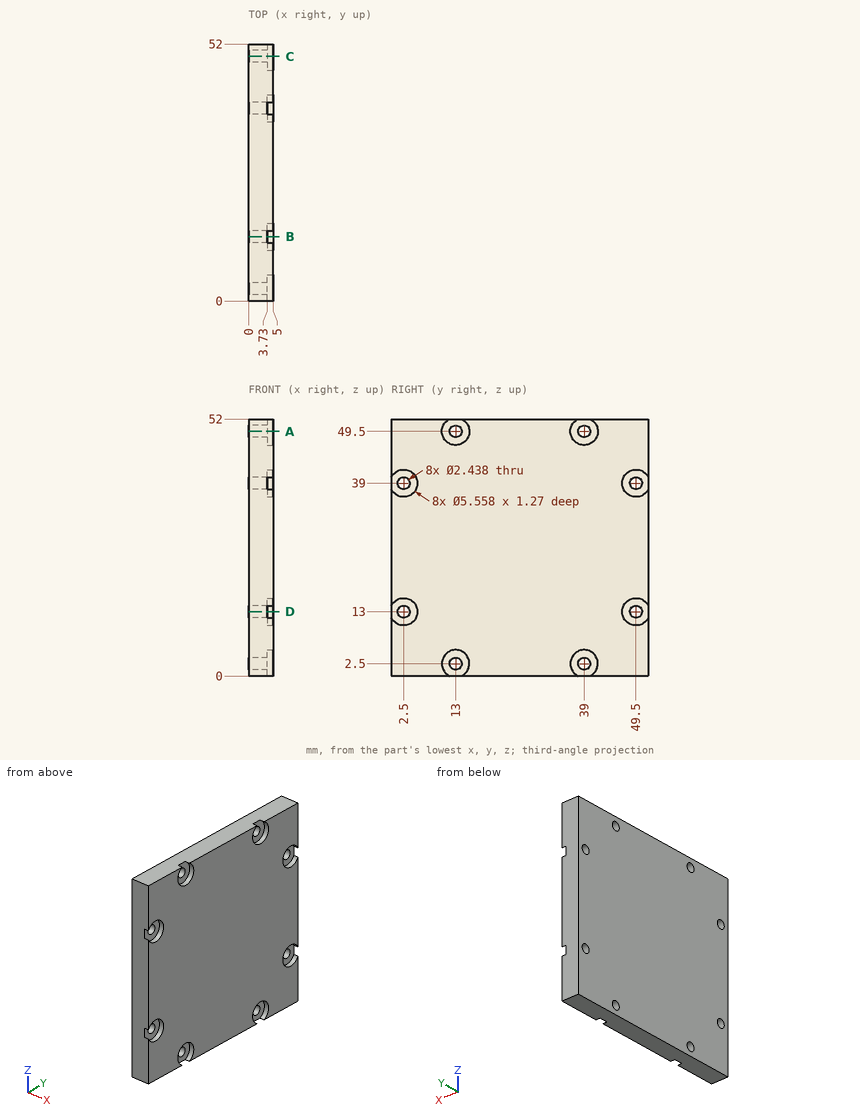
Drawing for the job (mm, zero at the part's lowest x, y, z). Give positions to 0.01 mm unless a question says otherwise; leave off trailing zeros. Order: outer loops, then holes, each group sorted by start corner. A loop starts at its lowest first (then second) coordinate and runs counter-clockwise, first axis right, second up. Notation, with made-up numbers: M 18,37 L 44,37 A6 ccw 44,48 Z; hole C -24,35 d8. An arc over 180 degrees is marked long. Put each result on its own line as item: value.
Item 1: Probe line 1 (Y direction, x = 1.1, z = 49.5); line 2 (Y direction, x = 4.3, z = 36.5) (1 decimal); line 3 (Z direction, x = 4.7, y = 2.5). List the from-to ranges inside material, lowest first. Write a range as [from, to].
From the geometry:
line 1: y = [0, 11.78], [14.22, 37.78], [40.22, 52]
line 2: y = [0, 1.3], [3.7, 48.3], [50.7, 52]
line 3: z = [0, 10.22], [15.78, 36.22], [41.78, 52]
Item 2: Flat gauge pins, fed straight in: pin 1 Ø3 at (y, z) = (13, 2.5) entering from +X; pin 2 Ø6 at (y, z) = (14.5, 30.5) entering from -X; pin 3 Ø2 at (y, z) = (2.5, 39) entering from -X. Where does each tip first touch, or does it go through?
From the geometry:
pin 1: stops at x = 3.73
pin 2: stops at x = 0
pin 3: passes through
Item 3: Slice it at B-B, the plane y = 13. Write the cut outline in (x, z).
From the geometry:
outline: M 0,0 L 3.73,0 L 3.73,1.28 L 0,1.28 Z; M 0,3.72 L 3.73,3.72 L 3.73,5.28 L 5,5.28 L 5,46.72 L 3.73,46.72 L 3.73,48.28 L 0,48.28 Z; M 0,50.72 L 3.73,50.72 L 3.73,52 L 0,52 Z
Item 4: Slice it at A-A, the plane z = 49.5. Write the cut outline in (x, y), plus the area to 3 significant figures.
From the geometry:
outline: M 0,0 L 5,0 L 5,10.22 L 3.73,10.22 L 3.73,11.78 L 0,11.78 Z; M 0,14.22 L 3.73,14.22 L 3.73,15.78 L 5,15.78 L 5,36.22 L 3.73,36.22 L 3.73,37.78 L 0,37.78 Z; M 0,40.22 L 3.73,40.22 L 3.73,41.78 L 5,41.78 L 5,52 L 0,52 Z
area: 228 mm2
